The listing builds one solid part. Answer for the finished solid, in the listing's coordinates (mm). Face numbers are marked on the shaded views. A direction names the side the tool comes from. Round coordinates to 2 decimals unless told otherwise and drop trailing zeros. Loops run counter-clockwise (first coordinate to the right, second up) from the corner with the lowest first, then second, coordinate; pieces in that order, holes last. Notation, with made-up numbers: (57, 85.25) -> (82, 85.25) arc R16 ccw to (82, 100.25) -> close; hole circle Ø7 at (73, 15). An arc over 180 degrees is marked (long way). Write each question's results on one line, items separated by ' | '. Start each with the question number.
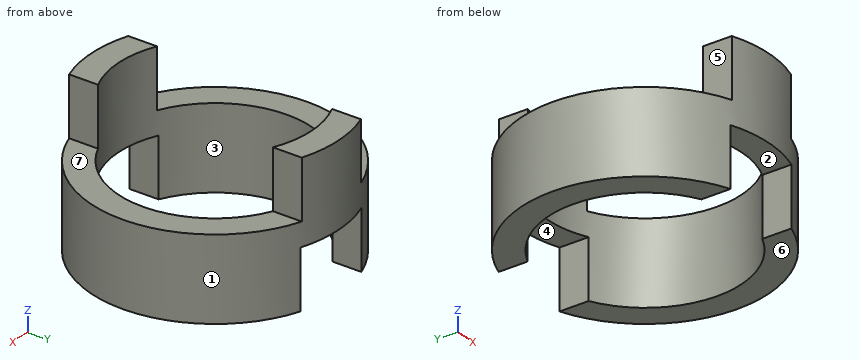
Autodesk Fusion 360 part; units mm, degrees
sketch "Sketch1" plane through (0, 0, 0) normal (0, 0, 1) x (1, 0, 0)
  circle A0 centre (0, 0) radius 5.25
  circle A1 centre (0, 0) radius 4.1
  dimension "d1" = 10.5
  dimension "d2" = 8.2
extrude "Extrude1" add sketch "Sketch1" along normal blind 6
sketch "Sketch2" plane through (0, 0, 0) normal (0, 0, -1) x (1, 0, 0)
  circle A0 centre (0, 0) radius 4.1
  circle A1 centre (0, 0) radius 5.25
  line L0 (-1.75, 6.7486) -> (1.75, 6.7486)
  line L1 (1.75, 6.7486) -> (1.75, -6.7486)
  line L2 (1.75, -6.7486) -> (-1.75, -6.7486)
  line L3 (-1.75, -6.7486) -> (-1.75, 6.7486)
  line L4 (-1.75, 6.7486) -> (1.75, -6.7486) construction
  line L5 (1.75, 6.7486) -> (-1.75, -6.7486) construction
  dimension "d5" = 3.5
extrude "Extrude2" cut sketch "Sketch2" against normal blind 2.5 contours A0 A1 L1 L3 | A0 A1 L1 L3
sketch "Sketch3" plane through (0, 0, 6) normal (0, 0, 1) x (-1, 0, 0)
  circle A0 centre (0, 0) radius 4.1
  circle A1 centre (0, 0) radius 5.25
  line L0 (-1.7, -5.9064) -> (1.7, -5.9064)
  line L1 (1.7, -5.9064) -> (1.7, 5.9064)
  line L2 (1.7, 5.9064) -> (-1.7, 5.9064)
  line L3 (-1.7, 5.9064) -> (-1.7, -5.9064)
  line L4 (-1.7, -5.9064) -> (1.7, 5.9064) construction
  line L5 (1.7, -5.9064) -> (-1.7, 5.9064) construction
  dimension "d8" = 3.4
extrude "Extrude3" cut sketch "Sketch3" against normal blind 2.5 contours A0 A1 L1 | A0 A1 L3
Item 1: For the marked faces 4, 5, 6 and 7, determine the directions among +Z, -Z, +X, -X, +Y, -Y from which every point of the face is accessible in a straight line to the end or side of a thin tool.
Item 2: Each of these flat-tipped pins is pushed along its axis until it touches: pin 1 Ø1.8 at (x, y) = (-3, 1.5) entering from +Z; pin 2 Ø2 at (x, z) = (-3, 0.5) entering from +Y; pin 3 Ø1 at (y, z) = (-4, 1.5) entering from +X. Where does it stop, or does it pass through?
Item 3: Straight lines are drawn through the part: L1, parallel to X at y = 0, z = 3.1; L2, parallel to Z at x = -4.5, y = 1.5. For each, find the intervals that lie inside material, in ascending order. Write a range as [from, to].
Item 4: The part is cut by section A-A, the plane z = 5.05. Give the vertices of the cut face in (x, y).
Item 5: The part is cut by section B-B, the plane x = 0. Give the vertices of the cut face in (y, z), plus the area to 3 significant figures.
Item 6: Determine the mould class of the marked faces 1, 2 and 3 for opening direction Y: +Y half, -Y half, draft (parallel to the pull), parting line (faces both ways), or undercut.
Report:
1) face 4: -Z, +Y, -Y | face 5: +Z, -X, +Y, -Y | face 6: -Z, +X, -X, +Y, -Y | face 7: +Z, +X, +Y, -Y
2) pin 1: stops at z = 3.5 | pin 2: stops at y = 4.85 | pin 3: stops at x = 3.91
3) L1: x = [-5.25, -4.1], [4.1, 5.25] | L2: z = [0, 3.5]
4) outline: (-1.7, -4.97) arc R5.25 ccw to (1.7, -4.97) -> (1.7, -3.73) arc R4.1 cw to (-1.7, -3.73) -> close; (-1.7, 3.73) arc R4.1 cw to (1.7, 3.73) -> (1.7, 4.97) arc R5.25 ccw to (-1.7, 4.97) -> close
5) outline: (-5.25, 2.5) -> (-4.1, 2.5) -> (-4.1, 6) -> (-5.25, 6) -> close; (4.1, 2.5) -> (5.25, 2.5) -> (5.25, 6) -> (4.1, 6) -> close | area: 8.05 mm2
6) face 1: parting line | face 2: draft | face 3: undercut
